Work out the finished part from the listing and answer in its coordinate system (mm). A direction names the side the tool comes from. Give positions to 0.01 mm unless a question says otherwise; leave off trailing zeros. Loops run counter-clockwise (first coordinate to the right, second up) from the corner with the lowest first, then second, coordinate; pieces in that order, holes last. Notation, with made-up numbers: M 13,41.25 L 41,41.25 A17 cw 41,63.25 Z; hole C 74,52.25 d9. An arc over 180 degrees is marked long. Write item = value, one per line. Start each with the question number.
1. For faces 4 (the face through (16.684, 3.972, -6.798)), 5 (the face through (18.376, 5.903, -0.034)), 6 (the face through (6.798, 3.972, 16.684)), 7 (the face through (-7, 2, -17)), 8 (the face through (-7, 4, 16.6)), determine the directions among +Z, -Z, +X, -X, +Y, -Y from which every point of the face is accessible in a straight line to the end or side of a thin tool.
2. Section A-A on y = 3.55 is taken. Determine the outline of the cut face in (x, z), plus the area to 3 significant figures.
3. Consider L1, parallel to Z at x = 0, y = 2.45; L2, parallel to X at y = 1.1, z = -0.5; L3, parallel to X at y = 4.4, z = -10.5. Determine where each line is inside the solid, lowest interval first. Write a range as [from, to].
4. The mould has two halves that part along Z. Classify faces 1 (the face through (-16.684, 3.972, 6.798)), 2 (the face through (2.539, 0.986, -19.334)), 3 (the face through (-12.5, 3.04, 3.94)): released by +Z, released by -Z, zero draft, split by the parting line, or undercut.
5. Flat-ended cylindrical pins translate along their axes: pin 1 Ø3 at (y, z) = (0.5, 9) entering from -X; pin 2 Ø6.5 at (x, z) = (-16, -10) entering from +Y; pin 3 Ø1.5 at (x, y) = (11, 4.5) entering from +Z; pin 4 Ø1.5 at (x, y) = (9, 1.5) entering from +Z. Find the tip coordinate at first contact, or state that the pin passes through.
6. Section B-B on y = 1.45 is taken. Determine the outline of the cut face in (x, z), plus the area to 3 significant figures.
Autodesk Inventor part; units mm, degrees
ref_plane "nut_body_XY" through (0, 0, 0) normal (0, -1, 0) x (1, 0, 0)
ref_plane "nut_body_YZ" through (0, 0, 0) normal (1, 0, 0) x (0, 0, 1)
ref_plane "nut_body_ZX" through (0, 0, 0) normal (0, 0, 1) x (0, -1, 0)
sketch "Sketch_1" plane through (0, 0, 0) normal (0, 0, 1) x (1, 0, 0)
  line L0 (0, 4) -> (0, 0)
  line L1 (-23.4, 4.5573) -> (-23.4, 2)
  line L2 (-23.4, 2) -> (-19.5, 2)
  line L3 (-19.5, 2) -> (-19.5, 0)
  line L4 (-19.5, 0) -> (-13.1055, 0)
  line L5 (-13.1055, 0) -> (-13.1055, 6)
  line L6 (-13.1055, 6) -> (-18.0157, 6)
  line L7 (-18.0157, 6) -> (-23.4, 4.5573)
revolve "Revolution1" add sketch "Sketch_1" angle 360 about axis through (0, 4, 0) along (0, 1, 0)
thread "Thread1"
sketch "Sketch_4" plane through (0, 2, 0) normal (0, 1, 0) x (1, 0, 0)
  circle A0 centre (0, 0) radius 50
  line L0 (-19.5, 0) -> (-13.7886, -13.7886)
  line L1 (-13.7886, -13.7886) -> (0, -19.5)
  line L2 (0, -19.5) -> (13.7886, -13.7886)
  line L3 (13.7886, -13.7886) -> (19.5, 0)
  line L4 (19.5, 0) -> (13.7886, 13.7886)
  line L5 (13.7886, 13.7886) -> (0, 19.5)
  line L6 (0, 19.5) -> (-13.7886, 13.7886)
  line L7 (-13.7886, 13.7886) -> (-19.5, 0)
extrude "Extrusion1" cut sketch "Sketch_4" along normal blind 4
ref_plane "nut_body_XY" through (0, 0, 0) normal (0, -1, 0) x (1, 0, 0)
ref_plane "nut_body_YZ" through (0, 0, 0) normal (1, 0, 0) x (0, 0, 1)
ref_plane "nut_body_ZX" through (0, 0, 0) normal (0, 0, 1) x (0, -1, 0)
properties part number "AP100_30_NUT"
Verdict:
q1.face_4 = -Z, +X, +Y
q1.face_5 = +X, +Y
q1.face_6 = +Z, +X, +Y
q1.face_7 = -Z, -X, +Y
q1.face_8 = +Z, -X, +Y
q2.outline = M -19.5,0 L -13.79,-13.79 L 0,-19.5 L 13.79,-13.79 L 19.5,0 L 13.79,13.79 L 0,19.5 L -13.79,13.79 Z; hole C 0,0 d26.21
q2.area = 536 mm2
q3.L1 = [-19.5, -13.11], [13.11, 19.5]
q3.L2 = [-19.49, -13.1], [13.1, 19.49]
q3.L3 = [-15.15, -7.84], [7.84, 15.15]
q4.face_1 = released by +Z
q4.face_2 = split by the parting line
q4.face_3 = undercut
q5.pin_1 = -18
q5.pin_2 = 6
q5.pin_3 = 15.25
q5.pin_4 = 17.67
q6.outline = C 0,0 d39; hole C 0,0 d26.21
q6.area = 655 mm2
